```python
from build123d import *

# Parameters (mm, degrees)
BOSS_EXTRUDE1_DEPTH      = 2.5
BOSS_EXTRUDE2_DEPTH      = 1.5
BOSS_EXTRUDE2_DEPTH_BACK = 1.5
FILLET1_R                = 1.5
SKETCH5_W                = 9.8
SKETCH5_H                = 10
BOSS_EXTRUDE3_DEPTH      = 7.5
SKETCH6_R                = 2.55
CUT_EXTRUDE1_DEPTH       = 8
FILLET2_R                = 3
SKETCH8_R                = 3
SKETCH8_R_2              = 2.6
BOSS_EXTRUDE4_DEPTH      = 0.8
SKETCH9_W                = 0.75667274
SKETCH9_H                = 5.4
CUT_EXTRUDE3_DEPTH       = 3
SKETCH10_R               = 3
CUT_EXTRUDE4_DEPTH       = 3
CUT_EXTRUDE5_DEPTH       = 10


with BuildPart() as part:
    # Sketch1 → Boss-Extrude1 (new body)
    with BuildSketch(Plane(origin=(0, 0, 0), x_dir=(1, 0, 0), z_dir=(0, 1, 0))):
        with BuildLine():
            Line((-20.209371097, 50.622586501), (-32.257467167, 50.622586501))
            ThreePointArc((-32.257467167, 50.622586501), (-33.362688598, 43.122586501), (-32.257467167, 35.622586501))
            Line((-32.257467167, 35.622586501), (-20.209371097, 35.622586501))
            Line((-20.209371097, 35.622586501), (-12.362688598, 37.872586501))
            Line((-12.362688598, 37.872586501), (-12.362688598, 48.372586501))
            Line((-12.362688598, 48.372586501), (-20.209371097, 50.622586501))
        make_face()
        with BuildLine():
            Line((-32.257467167, 50.622586501), (-34.339530518, 50.622586501))
            ThreePointArc((-34.339530518, 50.622586501), (-35.362688598, 43.122586501), (-34.339530518, 35.622586501))
            Line((-34.339530518, 35.622586501), (-32.257467167, 35.622586501))
            ThreePointArc((-32.257467167, 35.622586501), (-33.362688598, 43.122586501), (-32.257467167, 50.622586501))
        make_face()
    extrude(amount=BOSS_EXTRUDE1_DEPTH)

    # Sketch4 → Boss-Extrude2 (add, two sides)
    with BuildSketch(Plane.XZ) as boss_extrude2_sk:
        with BuildLine():
            Line((-19.362688598, -38.122586501), (-32.877390242, -38.122586501))
            ThreePointArc((-32.877390242, -38.122586501), (-33.362688598, -43.122586501), (-32.877390242, -48.122586501))
            Line((-32.877390242, -48.122586501), (-19.362688598, -48.122586501))
            Line((-19.362688598, -48.122586501), (-19.362688598, -38.122586501))
        make_face()
    extrude(amount=BOSS_EXTRUDE2_DEPTH)
    extrude(boss_extrude2_sk.sketch, amount=-BOSS_EXTRUDE2_DEPTH_BACK)

    # Fillet1
    fillet1_edges = [part.edges().sort_by_distance(p)[0] for p in [
        (-27.274450808, 2.5, -35.622586501),
        (-16.286029847, 2.5, -36.747586501),
        (-12.362688598, 2.5, -43.122586501),
        (-16.286029847, 2.5, -49.497586501),
        (-27.274450808, 2.5, -50.622586501),
        (-35.362688598, 2.5, -43.122586501),
    ]]
    fillet(fillet1_edges, radius=FILLET1_R)

    # Sketch5 → Boss-Extrude3 (add)
    with BuildSketch(Plane.XZ.offset(1.5)):
        with Locations((-24.262688598, -43.122586501)):
            Rectangle(SKETCH5_W, SKETCH5_H)
    extrude(amount=BOSS_EXTRUDE3_DEPTH)

    # Sketch6 → Cut-Extrude1 (cut)
    with BuildSketch(Plane(origin=(-19.362688598, 0, 0), x_dir=(0, 0, -1), z_dir=(1, 0, 0))):
        with Locations((43.122586501, -5.5)):
            Circle(SKETCH6_R)
    extrude(amount=-CUT_EXTRUDE1_DEPTH, mode=Mode.SUBTRACT)

    # Fillet2
    fillet2_edges = [part.edges().sort_by_distance(p)[0] for p in [
        (-24.262688598, -9, -38.122586501),
        (-24.262688598, -9, -48.122586501),
    ]]
    fillet(fillet2_edges, radius=FILLET2_R)

    # Sketch8 → Boss-Extrude4 (add)
    with BuildSketch(Plane.ZY.offset(29.162688598)):
        with Locations((-43.122586501, -5.5)):
            Circle(SKETCH8_R)
        with Locations((-43.122586501, -5.5)):
            Circle(SKETCH8_R_2, mode=Mode.SUBTRACT)
    extrude(amount=-BOSS_EXTRUDE4_DEPTH)

    # Sketch9 → Cut-Extrude3 (cut)
    with BuildSketch(Plane(origin=(0, -9, 0), x_dir=(-1, 0, 0), z_dir=(0, -1, 0))):
        with Locations((28.784352228, 43.122586501)):
            Rectangle(SKETCH9_W, SKETCH9_H)
    extrude(amount=-CUT_EXTRUDE3_DEPTH, mode=Mode.SUBTRACT)

    # Sketch10 → Cut-Extrude4 (cut)
    with BuildSketch(Plane(origin=(-27.362688598, 0, 0), x_dir=(0, 0, -1), z_dir=(1, 0, 0))):
        with Locations((43.122586501, -5.5)):
            Circle(SKETCH10_R)
    extrude(amount=-CUT_EXTRUDE4_DEPTH, mode=Mode.SUBTRACT)

    # Sketch11 → Cut-Extrude5 (cut)
    with BuildSketch(Plane.XZ):
        with BuildLine():
            Line((-19.362688598, -38.122586501), (-32.877390242, -38.122586501))
            ThreePointArc((-32.877390242, -38.122586501), (-33.362688598, -43.122586501), (-32.877390242, -48.122586501))
            Line((-32.877390242, -48.122586501), (-19.362688598, -48.122586501))
            Line((-19.362688598, -48.122586501), (-19.362688598, -38.122586501))
        make_face()
        with BuildLine():
            Line((-19.612688598, -38.372586501), (-32.670790068, -38.372586501))
            ThreePointArc((-32.670790068, -38.372586501), (-33.112688598, -43.122586501), (-32.670790068, -47.872586501))
            Line((-32.670790068, -47.872586501), (-19.612688598, -47.872586501))
            Line((-19.612688598, -47.872586501), (-19.612688598, -38.372586501))
        make_face(mode=Mode.SUBTRACT)
    extrude(amount=CUT_EXTRUDE5_DEPTH, mode=Mode.SUBTRACT)


solid = part.part
```
Could you check a few things on this model? Use its own coordinates, in mm. A direction names the side the tool comes from. Give positions to 0.01 mm unless a question says otherwise; leave off trailing zeros. Loops run counter-clockwise (first coordinate to the right, second up) from the corner with the lowest first, then second, coordinate; pieces in that order, holes last. Notation, with made-up numbers: (14, -36) - (43, -36) arc R25 ccw to (43, -6) - close; hole circle Ø7 at (25.5, -37). An arc over 180 degrees is marked (long way). Use one line per item in the form item = value.
1. I want a section at B-B (x = -30.25). Please give me the cut outline in (y, z), and give its area (3 significant figures).
Response values:
outline = (-1.5, -47.87) - (0, -47.87) - (0, -50.62) - (1, -50.62) arc R1.5 ccw to (2.5, -49.12) - (2.5, -37.12) arc R1.5 ccw to (1, -35.62) - (0, -35.62) - (0, -38.37) - (-1.5, -38.37) - close
area = 50.8 mm²
2. I want a section at D-D (y = 0.75). Please give me the cut outline in (x, z), and give its area (3 significant figures).
Response values:
outline = (-34.34, -50.62) - (-20.21, -50.62) - (-12.36, -48.37) - (-12.36, -37.87) - (-20.21, -35.62) - (-34.34, -35.62) arc R28 ccw to start
area = 322 mm²
3. I want a section at C-C (x = -21). Please give me the cut outline in (y, z), and give its area (3 significant figures).
Response values:
outline = (-9, -45.12) arc R3 ccw to (-7.2, -47.87) - (0, -47.87) - (0, -50.62) - (1, -50.62) arc R1.5 ccw to (2.5, -49.12) - (2.5, -37.12) arc R1.5 ccw to (1, -35.62) - (0, -35.62) - (0, -38.37) - (-7.2, -38.37) arc R3 ccw to (-9, -41.12) - close; hole circle Ø5.1 at (-5.5, -43.12)
area = 98.8 mm²
4. I'm going to push flat-ended pins straight in: pin 1 Ø0.8 at (x, y) = (-29, -8.5) entering from -Z (3 decimals); pin 2 Ø2 at (x, z) = (-32, -42) entering from -Y; pin 3 Ø5 at (x, y) = (-28.5, -5) entering from +Z. Where does each tip first touch, or does it pass through?
Response values:
pin_1 = -47.265
pin_2 = -1.5
pin_3 = -38.37
5. On a 3-axis mill with a long thin cutter (end or side, diameter ignored), from which of +Z, -Z, +X, -X, +Y, -Y can I reach the whole of each face in a straight line? I mean faces 4 (the face through (-25, -4, -38.373)), 5 (the face through (-16.23, 0.49, -49.48)), 6 (the face through (-31, -1.5, -43)). Say none if no direction works.
Response values:
face_4 = +Z, +X, -X, -Y
face_5 = -Z, +X, +Y, -Y
face_6 = +Z, -Z, -X, -Y
6. I want a section at A-A (y = -5.5). Please give me the cut outline in (x, z), and give its area (3 significant figures).
Response values:
outline = (-29.16, -47.87) - (-19.61, -47.87) - (-19.61, -45.67) - (-27.36, -45.67) - (-27.36, -46.12) - (-29.16, -46.12) - close; (-29.16, -40.12) - (-27.36, -40.12) - (-27.36, -40.57) - (-19.61, -40.57) - (-19.61, -38.37) - (-29.16, -38.37) - close
area = 40.4 mm²
7. Thinking about a two-plate mould opening in Y: for faces 1 (the face through (-24.321, -8.496, -46.787)), 2 (the face through (-23.433, -5.388, -40.575)), 3 (the face through (-16.341, 0.493, -36.732)), which applies, released by +Y, released by -Y, zero draft, split by the parting line, or undercut?
Response values:
face_1 = released by -Y
face_2 = undercut
face_3 = zero draft
8. I need wall thicknesses on probe 1 along Z at (x, y) = (-28.4, -5.5); probe 2 along Y at (x, z) = (-18, -44.75); probe 3 along Y at (x, z) = (-30, -45.5). Which ranges of each line are inside material? Lowest first, please.
Response values:
probe_1 = -47.87 to -46.12, -40.12 to -38.37
probe_2 = 0 to 2.5
probe_3 = -1.5 to 2.5
